Build history of the part. All positions in model axes, mm. A direction names the side the tool comes from. Round coordinates to 2 decimals unless told otherwise and drop trailing zeros. Write each loop counter-clockwise with the first axis right and the second up, starting at its lowest first coordinate (ties: lowest second). Pieces come first, ordered by that corner, then holes.
Item 1: Drop flat-ended pins along their axis: pin 1 Ø1.4 at (x, y) = (3.5, 37) entering from +Z; pin 2 Ø1 at (x, y) = (2, 11.5) entering from -Z; pin 3 Ø2.5 at (x, y) = (2, 13.5) entering from +Z. Give the stop position or say it passes through.
Item 2: 3-axis set-ups, long thin cutter, end or side, ignore diameter. For faces 1 (the flat face through (3, 15, 4)), 2 (the cylindrical face through (2.15, 40.44, 4.74)), 3 (the flat face through (4, 10.7, 22)): which of +Z, -Z, +X, -X, +Y, -Y reach the whole face in a straight line?
Item 3: Wall check: probe 1 along X at (y, z) = (40.5, 6.75); probe 2 along Y at (x, z) = (3.75, 6); probe 3 along Y at (x, z) = (3.5, 3). Give the ranges that are in metal, low to high.
Item 4: Mould opens along Y. For faces 4 (the flat face through (3, 33, 4)), 5 (the cylindrical face through (0.57, 0.69, 35.03)), 6 (the flat face through (4, 36, 13)), 7 (the flat face through (7, 11, 17)) say: +Y half, -Y half, draft (parallel to the pull), parting line (faces both ways), or undercut.
Item 5: Band-saw the part on A-A, the plane z = 27. Write the cut outline in (x, y).
Autodesk Fusion 360 part; units mm, degrees
sketch "Sketch1" plane through (0, 0, 0) normal (0, 0, 1) x (1, 0, 0)
  line L0 (0, 0) -> (7, 0)
  line L1 (7, 0) -> (7, 48)
  line L2 (7, 48) -> (0, 48)
  line L3 (0, 48) -> (0, 0)
  circle A0 centre (3.5, 40.5) radius 1.35
  circle A1 centre (3.5, 7.5) radius 1.35
  line L4 (0, 33) -> (7, 33)
  line L5 (0, 15) -> (7, 15)
  dimension "d1" = 7
  dimension "d2" = 48
  dimension "d3" = 2.7
  dimension "d4" = 2.7
  dimension "d5" = 3.5
  dimension "d6" = 3.5
  dimension "d7" = 33
  dimension "d8" = 7.5
  dimension "d9" = 15
  dimension "d10" = 15
extrude "Extrude1" add sketch "Sketch1" along normal blind 13 contours L0 L1 L3 L5 | L1 L2 L3 L4 makes body 1 at (0, 10, 4.3333) makes body 2 at (0, 43, 4.3333)
extrude "Extrude2" add sketch "Sketch1" along normal blind 30 from surface at 9 contours L0 L1 L3 L5 | L1 L3 L4 L5 | L1 L2 L3 L4 | A0 | A1 bodies 1 2
sketch "Sketch2" plane through (7, 0, 0) normal (1, 0, 0) x (0, 1, 0)
  line L0 (33, 0) -> (48, 0)
  line L1 (48, 0) -> (48, 39)
  line L2 (48, 39) -> (0, 39)
  line L3 (0, 39) -> (0, 0)
  line L4 (0, 0) -> (15, 0)
  line L5 (15, 0) -> (15, 9)
  line L6 (15, 9) -> (33, 9)
  line L7 (33, 9) -> (33, 0)
  line L8 (12, 30.3) -> (36, 30.3)
  line L9 (36, 30.3) -> (36, 6.3)
  line L10 (36, 6.3) -> (12, 6.3)
  line L11 (12, 6.3) -> (12, 30.3)
  line L12 (0, 0) -> (48, 0)
  line L13 (12, 24.3) -> (10.7, 24.3)
  line L14 (10.7, 24.3) -> (10.7, 19.7)
  line L15 (10.7, 19.7) -> (12, 19.7)
  line L16 (12, 19.7) -> (12, 24.3)
  line L17 (36, 24.3) -> (37.3, 24.3)
  line L18 (37.3, 24.3) -> (37.3, 19.7)
  line L19 (37.3, 19.7) -> (36, 19.7)
  line L20 (36, 19.7) -> (36, 24.3)
  dimension "d18" = 24
  dimension "d19" = 24
  dimension "d20" = 12
  dimension "d22" = 6.3
  dimension "d31" = 6
  dimension "d32" = 6
  dimension "d33" = 4.6
  dimension "d34" = 4.6
  dimension "d35" = 1.3
  dimension "d36" = 1.3
extrude "Extrude3" cut sketch "Sketch2" against normal blind 7 contours L5 L6 L7 L10 | L5 L6 L7 L8 L9 L10 L11 L16 L20 | L9 L17 L18 L19 L20 | L11 L13 L14 L15 L16 bodies 1
fillet "Fillet3" radius 5 2 edges at (7, 48, 19.5) (7, 0, 19.5) on bodies 1
sketch "Sketch3" plane through (0, 48, 0) normal (0, 1, 0) x (-1, 0, 0)
  line L0 (-2, 39) -> (-2, 0)
  line L1 (-2, 0) -> (0, 0)
  line L2 (0, 0) -> (0, 39)
  line L3 (0, 0) -> (-7.1424, 2)
  line L4 (-7.1424, 2) -> (-7.1424, 0)
  line L5 (-7.1424, 0) -> (0, 0)
  line L6 (0, 39) -> (-2, 39)
  dimension "d39" = 2
fillet "Fillet4" radius 7 5 edges at (1, 0, 39) (5.5355, 1.4645, 39) (7, 24, 39) (5.5355, 46.5355, 39) (1, 48, 39) on bodies 1
extrude "Extrude4" cut sketch "Sketch3" against normal blind 50 contours L0 L1 L3 L5 | L0 L3 L4 L5 bodies 1
fillet "Fillet2" [suppressed]
equation "d14 = 28.00 mm + 2 mm"
Results:
1. pin 1: stops at z = 38.42
1. pin 2: stops at z = 0.42
1. pin 3: stops at z = 38.96
2. face 1: -Z, +X, -X
2. face 2: -Z
2. face 3: +X, -X
3. probe 1: x = 0 to 2.15, 4.85 to 7
3. probe 2: y = 0.32 to 6.17, 8.83 to 15, 33 to 39.17, 41.83 to 47.68
3. probe 3: y = 0.23 to 6.15, 8.85 to 15, 33 to 39.15, 41.85 to 47.77
4. face 4: undercut
4. face 5: -Y half
4. face 6: undercut
4. face 7: draft
5. outline: (0, 0) - (2, 0) arc R5 ccw to (7, 5) - (7, 12) - (0, 12) - close; (0, 36) - (7, 36) - (7, 43) arc R5 ccw to (2, 48) - (0, 48) - close
